Autodesk Inventor part; units mm, degrees
ref_plane "YZ Plane" through (0, 0, 0) normal (1, 0, 0) x (0, 1, 0)
ref_plane "XZ Plane" through (0, 0, 0) normal (0, 1, 0) x (-1, 0, 0)
ref_plane "XY Plane" through (0, 0, 0) normal (0, 0, 1) x (1, 0, 0)
sketch "Sketch1" plane through (0, 0, 0) normal (0, 1, 0) x (-1, 0, 0)
  line L0 (0, 0) -> (-50, 0)
  line L1 (-50, 0) -> (-50, -50)
  line L2 (-50, -50) -> (0, -50)
  line L3 (0, -50) -> (0, 0)
  dimension "d0" = 50
  dimension "d1" = 50
extrude "Extrusion1" add sketch "Sketch1" along normal blind 55
sketch "Sketch2" plane through (0, 0, 0) normal (0, 0, 1) x (1, 0, 0)
  line L0 (0, 0) -> (50, 0)
  line L1 (45, 0) -> (45, 6)
  line L2 (50, 0) -> (50, 55)
  line L3 (5, 0) -> (5, 6)
  line L4 (0, 0) -> (0, 55)
  line L5 (5, 6) -> (45, 6)
  line L6 (5, 0) -> (45, 0)
  dimension "d7" = 6
  dimension "d8" = 5
  dimension "d9" = 5
sketch "Sketch3" plane through (0, 0, 0) normal (0, 0, 1) x (1, 0, 0)
  point P0 (0, 0)
sketch "Sketch4" plane through (0, 55, 0) normal (0, 1, 0) x (1, 0, 0)
  circle A0 centre (25, 25) radius 10.5
  line L0 (0, 50) -> (0, 0)
  line L1 (0, 0) -> (50, 0)
  dimension "d10" = 21
  dimension "d11" = 25
  dimension "d12" = 25
extrude "Extrusion2" cut sketch "Sketch2" against normal blind 55
extrude "Extrusion3" add sketch "Sketch4" along normal blind 20
sketch "Sketch5" plane through (50, 0, 0) normal (1, 0, 0) x (0, 0, -1)
  line L0 (50, 0) -> (8, 0)
  line L1 (0, 0) -> (50, 0)
  line L2 (8, 0) -> (8, 6)
  line L3 (0, 55) -> (50, 55)
  line L4 (50, 0) -> (50, 55)
  line L5 (50, 0) -> (50, 44)
  line L6 (8, 6) -> (50, 44)
  dimension "d17" = 42
  dimension "d18" = 6
  dimension "d27" = 44
extrude "Extrusion4" add sketch "Sketch5" along normal blind 40
sketch "Sketch6" plane through (50, 0, -8) normal (0, 0, 1) x (1, 0, 0)
  point P0 (-50, 0)
sketch "Sketch7" plane through (50, 6, -8) normal (0, 0.6987, 0.7154) x (1, 0, 0)
  point P0 (-50, -9.8822)
sketch "Sketch8" plane through (50, 6, -8) normal (0, 0.6987, 0.7154) x (1, 0, 0)
  point P0 (-50, -9.8822)
sketch "Sketch9" plane through (90, 0, 0) normal (1, 0, 0) x (0, 0, -1)
  line L0 (0, 0) -> (50, 0)
  line L1 (50, 0) -> (8, 0)
  line L2 (8, 0) -> (8, 47)
  line L3 (8, 47) -> (50, 47)
  line L4 (50, 47) -> (50, 0)
  dimension "d22" = 42
  dimension "d23" = 47
extrude "Extrusion5" add sketch "Sketch9" along normal blind 15
sketch "Sketch10" plane through (50, 0, -8) normal (0, 0, 1) x (1, 0, 0)
  point P0 (-50, 0)
sketch "Sketch11" plane through (50, 0, -8) normal (0, 0, 1) x (1, 0, 0)
  line L0 (40, 0) -> (26, 0)
  line L1 (26, 0) -> (26, 12)
  line L2 (26, 12) -> (40, 12)
  line L3 (40, 12) -> (40, 0)
  point P0 (-50, 0)
  dimension "d28" = 14
  dimension "d29" = 12
extrude "Extrusion6" cut sketch "Sketch11" against normal blind 11
properties part number "400185627_VD"
Here's how the part is built. I have some questions about the finished solid (model axes, mm). A direction names the side the tool comes from. Coordinates: 2 decimals unless noted, no trailing zeros. Order: outer loops, then holes, each group sorted by start corner. A loop starts at its lowest first (then second) coordinate and runs counter-clockwise, first axis right, second up.
Item 1: Which directions (+Z, -Z, +X, -X, +Y, -Y) give clear straight access to the entire face, cutting with the end or side of a thin tool? Please do faces 1 (the face through (83, 6, -19)), 2 (the face through (97, 47, -29)), 3 (the face through (17.261, 64.86, -17.904)), 4 (the face through (63, 3, -8)).
Response values:
face 1: +Z, -Y
face 2: +Z, -Z, +X, +Y
face 3: +Y
face 4: +Z, +X, +Y, -Y
Item 2: If we section it at D-D, the plane x = 83.5: List the corners of the cut face in (y, z) for me.
Response values:
outline: (0, -50) - (44, -50) - (12, -14.63) - (12, -19) - (0, -19) - close
Item 3: Thinking about a two-plate mould opening in X: for faces 5 (the face through (5, 3, -25)), 6 (the face through (25, 27, 0)), 7 (the face through (105, 24, -29)), which applies, pulls with the +X half, pulls with the -X half, needs draft (parallel to the pull), parting line crosses it, or undercut?
Response values:
face 5: undercut
face 6: needs draft
face 7: pulls with the +X half
Item 4: If we section it at B-B, the plane z = -5.5: List the corners of the cut face in (x, y) for me.
Response values:
outline: (0, 0) - (5, 0) - (5, 6) - (45, 6) - (45, 0) - (50, 0) - (50, 55) - (0, 55) - close
Item 5: If we section it at A-A, the plane x = 25: List the corners of the cut face in (y, z) for me, then the cut area to 3 significant figures.
Response values:
outline: (6, -50) - (55, -50) - (55, -35.5) - (75, -35.5) - (75, -14.5) - (55, -14.5) - (55, 0) - (6, 0) - close
area: 2,870 mm2
Item 6: If we section it at C-C, the plane y = 65.5: List the corners of the cut face in (x, z) for me.
Response values:
outline: circle Ø21 at (25, -25)
Item 7: I need wall thicknesses on probe 1 along X at (y, z) = (34.5, -37.5); probe 2 along X at (y, z) = (40.5, -6); probe 3 along Z at (x, y) = (72, 5.5). Which ranges of each line are inside material? Lowest first, please.
Response values:
probe 1: x = 0 to 50, 90 to 105
probe 2: x = 0 to 50
probe 3: z = -50 to -8
Item 8: I'm going to push flat-ended pins straight in: pin 1 Ø4.5 at (x, y) = (98, 18) entering from +Z; pin 2 Ø1.3 at (x, z) = (81, -16.5) entering from -Y; pin 3 Ø7.5 at (x, z) = (97.5, -39) entering from +Y. Where does each tip first touch, or does it pass through?
Response values:
pin 1: stops at z = -8
pin 2: stops at y = 12
pin 3: stops at y = 47
